```python
from build123d import *

# Parameters (mm, degrees)
EXTRUDE_1_DEPTH     = 10
SKETCH_2_R          = 3
CUT_EXTRUDE_1_DEPTH = 25


with BuildPart() as part:
    # Эскиз1 → Вытянуть1 (new body)
    with BuildSketch(Plane(origin=(0, 0, 0), x_dir=(0, 0, -1), z_dir=(1, 0, 0))):
        with BuildLine():
            Line((-19.99990009, 63.483695787), (-19.99990009, -30.143863535))
            Line((-19.99990009, -30.143863535), (20.00009991, -30.143863535))
            Line((20.00009991, -30.143863535), (20.00009991, 58.395614664))
            ThreePointArc((20.00009991, 58.395614664), (21.991555525, 67.095748523), (27.569332826, 74.063289338))
            ThreePointArc((27.569332826, 74.063289338), (30.358221476, 77.547059746), (31.353949284, 81.897126676))
            Line((31.353949284, 81.897126676), (31.353949284, 126.453197444))
            ThreePointArc((31.353949284, 126.453197444), (28.425017096, 133.524265256), (21.353949284, 136.453197444))
            Line((21.353949284, 136.453197444), (4.569303476, 136.453197444))
            ThreePointArc((4.569303476, 136.453197444), (-2.501764335, 133.524265256), (-5.430696524, 126.453197444))
            Line((-5.430696524, 126.453197444), (-5.430696524, 94.358841013))
            ThreePointArc((-5.430696524, 94.358841013), (-6.386997306, 90.091347082), (-9.072997415, 86.640054707))
            ThreePointArc((-9.072997415, 86.640054707), (-17.130997744, 76.286177582), (-19.99990009, 63.483695787))
        make_face()
    extrude(amount=EXTRUDE_1_DEPTH)

    # Эскиз2 → Вырез-Вытянуть1 (cut)
    with BuildSketch(Plane.ZY):
        with Locations((10, -22.643863535)):
            Circle(SKETCH_2_R)
        with Locations((-10, -22.643863535)):
            Circle(SKETCH_2_R)
        with Locations((-12.96162638, 126.453197444)):
            Circle(SKETCH_2_R)
    extrude(amount=-CUT_EXTRUDE_1_DEPTH, mode=Mode.SUBTRACT)


solid = part.part
```
The listing builds one solid part. Answer for the finished solid, in the listing's coordinates (mm). A direction names the side the tool comes from. Give positions to 0.01 mm unless a question says otherwise; leave off trailing zeros. Write each loop counter-clockwise with the first axis right and the second up, starting at its lowest first coordinate (ties: lowest second). Pieces come first, ordered by that corner, then holes. Notation, with made-up numbers: (71, -8) -> (95, -8) arc R26 ccw to (95, 23) -> close; hole circle Ø5 at (-25.5, 5). An arc over 180 degrees is marked (long way). Write item = value, one per line. Start each with the question number.
1) Which of the six approach directions +Z, -Z, +X, -X, +Y, -Y give full straight-line access (tool end or side, diameter ignored) to faces 1 (the face through (5, 136.453, -13)), 2 (the face through (5, 14, -20)), 3 (the face through (5, 111, 5.431))?
2) Determine the mould class of faces 4 (the face through (4.93, 66.982, -21.937)), 5 (the face through (4.93, -20.616, -12.211)), 6 (the face through (4.93, -20.114, 11.613)), 7 (the face through (4.93, 133.602, 2.424)) for opening direction Z: +Z half, -Z half, draft (parallel to the pull), parting line (faces both ways), or undercut.
3) Each of these flat-tipped pins is pushed along its axis until it touches: pin 1 (3 mm diameter, centred on x = 6, y = 13, fed in from -Z); pin 2 (5.5 mm diameter, centred on y = 126.45, z = -12.96, fed in from +X); pin 3 (6 mm diameter, centred on x = 9, z = 14, fed in from +Y). Where does it stop, or does it pass through?
4) Straight lines are drawn through the part: line 1 along Y through (x, z) = (4.75, 9); line 2 along Z through (x, y) = (8.75, 54); line 3 along Z through (x, y) = (7.25, 120). For each, find the intervals that lie inside material, in ascending order.
5) The part is cut by section C-C, the plane z = 3. Determine the outline of the cut face in (x, y), and give its area (3 significant figures).
6) The part is cut by section A-A, the plane x = 7.75. Determine the outline of the cut face in (y, z), and give its area (3 significant figures).
7) The part is cut by section B-B, the plane y = 2. Determine the outline of the cut face in (x, z).
Solutions:
q1.face_1 = +Z, -Z, +X, -X, +Y
q1.face_2 = -Z, +X, -X, -Y
q1.face_3 = +Z, +X, -X, +Y
q2.face_4 = -Z half
q2.face_5 = undercut
q2.face_6 = undercut
q2.face_7 = +Z half
q3.pin_1 = -20
q3.pin_2 = through
q3.pin_3 = 84.91
q4.line_1 = -30.14 to -25.47, -19.82 to 86.7
q4.line_2 = -20 to 20
q4.line_3 = -31.35 to 5.43
q5.outline = (0, -30.14) -> (10, -30.14) -> (10, 132.99) -> (0, 132.99) -> close
q5.area = 1,630 mm²
q6.outline = (-30.14, -20) -> (58.4, -20) arc R20 cw to (74.06, -27.57) arc R10 ccw to (81.9, -31.35) -> (126.45, -31.35) arc R10 ccw to (136.45, -21.35) -> (136.45, -4.57) arc R10 ccw to (126.45, 5.43) -> (94.36, 5.43) arc R10 cw to (86.64, 9.07) arc R30 ccw to (63.48, 20) -> (-30.14, 20) -> close; hole circle Ø6 at (-22.64, -10); hole circle Ø6 at (-22.64, 10); hole circle Ø6 at (126.45, -12.96)
q6.area = 6,480 mm²
q7.outline = (0, -20) -> (10, -20) -> (10, 20) -> (0, 20) -> close
